CAD build for the part. Positions are in the model's coordinates, mm. Face numbers are marked on the shaded views. A direction names the side the tool comes from. Give positions to 0.01 mm unless a question says otherwise; leave off trailing zeros. Order: outer loops, then holes, each group sorted by start corner. A loop starts at its lowest first (then second) coordinate and runs counter-clockwise, first axis right, second up. Notation, with made-up numbers: M -14,60 L -3,60 A23 ccw -3,96 Z; hole C -39.5,-33 d1. An arc over 180 degrees is marked long. Put each result on its own line as item: value. Start each with the question number.
1) Pin check, flat tips, straight feed: pin 1 (2.5 mm diameter, centred on x = 26, z = 0, fed in from -Y); pin 2 (10.5 mm diameter, centred on x = -23.5, z = 19.5, fed in from +Y); pin 3 (2.5 mm diameter, centred on x = -6.5, y = 1, fed in from +Z); pin 4 (2.5 mm diameter, centred on x = -5, y = 1.5, fed in from -Z). Stop position of each tip, or through.
2) Drill centre lines: line 1 (X direction, y = 9, z = 21); line 2 (Z direction, x = 22.5, y = 6.75); line 3 (X direction, y = 4, z = 12.5). Where is each one in solid material? Low to high. Write a range as [from, to].
3) Cut at C-C (z = -4.5). Write the cut outline in (x, y), and give its area (3 significant figures).
4) Cut at A-A (x = 26). Write the cut outline in (y, z), and give its area (3 significant figures).
5) Cut at D-D (y = 1.75). Write the cut outline in (x, z), and give its area (3 significant figures).
6) Cut at B-B (y = 7.75). Write the cut outline in (x, z), and give its area (3 significant figures).
7) Two-plate mould, pull along Z, no slides. Class the marked faces 1, 2, 3 and 4: released by +Z, released by -Z, zero draft, split by the parting line, or undercut.
8) Tool access for the marked faces 5, 6, 7 and 8: list every direction of +Z, -Z, +X, -X, +Y, -Y with a clear straight run to the whole face (end or side of a thin tool).
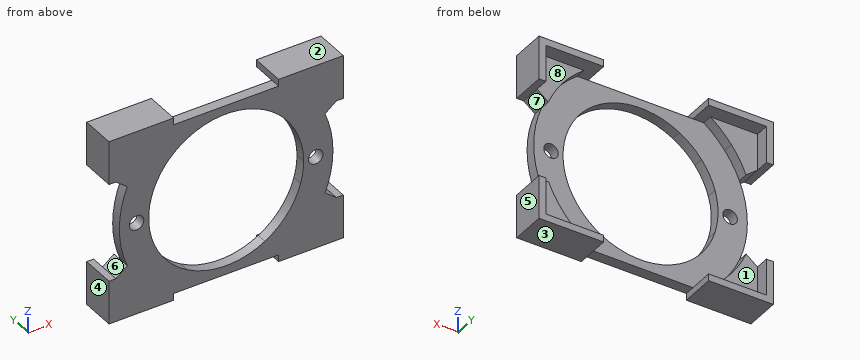
```python
from build123d import *

# Parameters (mm, degrees)
BOSS_EXTRUDE1_DEPTH   = 10
BOSS_EXTRUDE1_2_DEPTH = 10
BOSS_EXTRUDE1_3_DEPTH = 10
BOSS_EXTRUDE1_4_DEPTH = 10
SKETCH1_9_R           = 2.1
BOSS_EXTRUDE2_DEPTH   = 3
BOSS_EXTRUDE3_DEPTH   = 6


with BuildPart() as part:
    # Sketch1 → Boss-Extrude1 (new body)
    with BuildSketch(Plane(origin=(0, 0, 0), x_dir=(1, 0, 0), z_dir=(0, 1, 0))):
        Polygon((-15.231546212, -27), (-15.231546212, -25), (-18.33030278, -25), (-32, -25), (-32, -14.320549047), (-34, -14.320549047), (-34, -27), align=None)
    extrude(amount=BOSS_EXTRUDE1_DEPTH)



with BuildPart() as body_2:
    # Sketch1 → Boss-Extrude1 2 (new body)
    with BuildSketch(Plane(origin=(0, 0, 0), x_dir=(1, 0, 0), z_dir=(0, 1, 0))):
        Polygon((32, -14.320549047), (32, -25), (18.33030278, -25), (15.231546212, -25), (15.231546212, -27), (34, -27), (34, -14.320549047), align=None)
    extrude(amount=BOSS_EXTRUDE1_2_DEPTH)


with BuildPart() as body_3:
    # Sketch1 → Boss-Extrude1 3 (new body)
    with BuildSketch(Plane(origin=(0, 0, 0), x_dir=(1, 0, 0), z_dir=(0, 1, 0))):
        Polygon((32, 25), (32, 14.320549047), (34, 14.320549047), (34, 27), (15.231546212, 27), (15.231546212, 25), (18.33030278, 25), align=None)
    extrude(amount=BOSS_EXTRUDE1_3_DEPTH)


with BuildPart() as body_4:
    # Sketch1 → Boss-Extrude1 4 (new body)
    with BuildSketch(Plane(origin=(0, 0, 0), x_dir=(1, 0, 0), z_dir=(0, 1, 0))):
        Polygon((-18.33030278, 25), (-15.231546212, 25), (-15.231546212, 27), (-34, 27), (-34, 14.320549047), (-32, 14.320549047), (-32, 25), align=None)
    extrude(amount=BOSS_EXTRUDE1_4_DEPTH)


with BuildPart() as part_1:
    add(part.part)

    add(body_2.part)  # Boss-Extrude2 merges body 2

    add(body_3.part)  # Boss-Extrude2 merges body 3

    add(body_4.part)  # Boss-Extrude2 merges body 4
    # Sketch1_9 → Boss-Extrude2 (add)
    # profile 1 of 14: a face of its own
    with BuildSketch(Plane(origin=(0, 0, 0), x_dir=(1, 0, 0), z_dir=(0, 1, 0))):
        with BuildLine():
            Line((-32, 25), (-32, 14.320549047))
            Line((-32, 14.320549047), (-28.692414075, 11.736497543))
            ThreePointArc((-28.692414075, 11.736497543), (-24.428755585, 19.084965301), (-18.33030278, 25))
            Line((-18.33030278, 25), (-32, 25))
        make_face()
    # profile 2 of 14: a face of its own
    with BuildSketch(Plane(origin=(0, 0, 0), x_dir=(1, 0, 0), z_dir=(0, 1, 0))):
        with BuildLine():
            Line((-28.692414075, 11.736497543), (-21.624662992, 6.21481701))
            ThreePointArc((-21.624662992, 6.21481701), (-17.730548409, 13.851990944), (-11.262551698, 19.478319467))
            Line((-11.262551698, 19.478319467), (-18.33030278, 25))
            ThreePointArc((-18.33030278, 25), (-24.428755585, 19.084965301), (-28.692414075, 11.736497543))
        make_face()
    # profile 3 of 14: a face of its own
    with BuildSketch(Plane(origin=(0, 0, 0), x_dir=(1, 0, 0), z_dir=(0, 1, 0))):
        with BuildLine():
            Line((11.262551698, 19.478319467), (18.33030278, 25))
            Line((18.33030278, 25), (15.231546212, 25))
            Line((15.231546212, 25), (-15.231546212, 25))
            Line((-15.231546212, 25), (-18.33030278, 25))
            Line((-18.33030278, 25), (-11.262551698, 19.478319467))
            ThreePointArc((-11.262551698, 19.478319467), (0, 22.5), (11.262551698, 19.478319467))
        make_face()
    # profile 4 of 14: a face of its own
    with BuildSketch(Plane(origin=(0, 0, 0), x_dir=(1, 0, 0), z_dir=(0, 1, 0))):
        with BuildLine():
            Line((21.624662992, 6.21481701), (28.692414075, 11.736497543))
            ThreePointArc((28.692414075, 11.736497543), (24.428755585, 19.084965301), (18.33030278, 25))
            Line((18.33030278, 25), (11.262551698, 19.478319467))
            ThreePointArc((11.262551698, 19.478319467), (17.730548409, 13.851990944), (21.624662992, 6.21481701))
        make_face()
    # profile 5 of 14: a face of its own
    with BuildSketch(Plane(origin=(0, 0, 0), x_dir=(1, 0, 0), z_dir=(0, 1, 0))):
        with BuildLine():
            Line((28.692414075, 11.736497543), (32, 14.320549047))
            Line((32, 14.320549047), (32, 25))
            Line((32, 25), (18.33030278, 25))
            ThreePointArc((18.33030278, 25), (24.428755585, 19.084965301), (28.692414075, 11.736497543))
        make_face()
    # profile 6 of 14: a face of its own
    with BuildSketch(Plane(origin=(0, 0, 0), x_dir=(1, 0, 0), z_dir=(0, 1, 0))):
        with BuildLine():
            Line((21.624662992, -6.21481701), (28.692414075, -11.736497543))
            ThreePointArc((28.692414075, -11.736497543), (31, 0), (28.692414075, 11.736497543))
            Line((28.692414075, 11.736497543), (21.624662992, 6.21481701))
            ThreePointArc((21.624662992, 6.21481701), (22.280091083, 3.138079243), (22.5, 0))
            ThreePointArc((22.5, 0), (22.280091083, -3.138079243), (21.624662992, -6.21481701))
        make_face()
        with Locations(Location((26, 0, 0), (0, 0, 270))):
            Circle(SKETCH1_9_R, mode=Mode.SUBTRACT)
    # profile 7 of 14: a face of its own
    with BuildSketch(Plane(origin=(0, 0, 0), x_dir=(1, 0, 0), z_dir=(0, 1, 0))):
        with BuildLine():
            Line((-24.428755585, -19.084965301), (-17.730548409, -13.851990944))
            ThreePointArc((-17.730548409, -13.851990944), (-20.044694374, -10.220578627), (-21.624662992, -6.21481701))
            Line((-21.624662992, -6.21481701), (-28.692414075, -11.736497543))
            ThreePointArc((-28.692414075, -11.736497543), (-26.813516388, -15.557484979), (-24.428755585, -19.084965301))
        make_face()
    # profile 8 of 14: a face of its own
    with BuildSketch(Plane(origin=(0, 0, 0), x_dir=(1, 0, 0), z_dir=(0, 1, 0))):
        with BuildLine():
            Line((-28.692414075, -11.736497543), (-21.624662992, -6.21481701))
            ThreePointArc((-21.624662992, -6.21481701), (-22.5, 0), (-21.624662992, 6.21481701))
            Line((-21.624662992, 6.21481701), (-28.692414075, 11.736497543))
            ThreePointArc((-28.692414075, 11.736497543), (-31, 0), (-28.692414075, -11.736497543))
        make_face()
        with Locations(Location((-26, 0, 0), (0, 0, 270))):
            Circle(SKETCH1_9_R, mode=Mode.SUBTRACT)
    # profile 9 of 14: a face of its own
    with BuildSketch(Plane(origin=(0, 0, 0), x_dir=(1, 0, 0), z_dir=(0, 1, 0))):
        with BuildLine():
            Line((-32, -14.320549047), (-32, -25))
            Line((-32, -25), (-24.428755585, -19.084965301))
            ThreePointArc((-24.428755585, -19.084965301), (-26.813516388, -15.557484979), (-28.692414075, -11.736497543))
            Line((-28.692414075, -11.736497543), (-32, -14.320549047))
        make_face()
    # profile 10 of 14: a face of its own
    with BuildSketch(Plane(origin=(0, 0, 0), x_dir=(1, 0, 0), z_dir=(0, 1, 0))):
        with BuildLine():
            Line((-32, -25), (-18.33030278, -25))
            ThreePointArc((-18.33030278, -25), (-21.583122502, -22.252389154), (-24.428755585, -19.084965301))
            Line((-24.428755585, -19.084965301), (-32, -25))
        make_face()
    # profile 11 of 14: a face of its own
    with BuildSketch(Plane(origin=(0, 0, 0), x_dir=(1, 0, 0), z_dir=(0, 1, 0))):
        with BuildLine():
            Line((-18.33030278, -25), (-11.262551698, -19.478319467))
            ThreePointArc((-11.262551698, -19.478319467), (-14.766985359, -16.976046165), (-17.730548409, -13.851990944))
            Line((-17.730548409, -13.851990944), (-24.428755585, -19.084965301))
            ThreePointArc((-24.428755585, -19.084965301), (-21.583122502, -22.252389154), (-18.33030278, -25))
        make_face()
    # profile 12 of 14: a face of its own
    with BuildSketch(Plane(origin=(0, 0, 0), x_dir=(1, 0, 0), z_dir=(0, 1, 0))):
        with BuildLine():
            Line((15.231546212, -25), (18.33030278, -25))
            Line((18.33030278, -25), (11.262551698, -19.478319467))
            ThreePointArc((11.262551698, -19.478319467), (0, -22.5), (-11.262551698, -19.478319467))
            Line((-11.262551698, -19.478319467), (-18.33030278, -25))
            Line((-18.33030278, -25), (-15.231546212, -25))
            Line((-15.231546212, -25), (15.231546212, -25))
        make_face()
    # profile 13 of 14: a face of its own
    with BuildSketch(Plane(origin=(0, 0, 0), x_dir=(1, 0, 0), z_dir=(0, 1, 0))):
        with BuildLine():
            Line((11.262551698, -19.478319467), (18.33030278, -25))
            ThreePointArc((18.33030278, -25), (24.428755585, -19.084965301), (28.692414075, -11.736497543))
            Line((28.692414075, -11.736497543), (21.624662992, -6.21481701))
            ThreePointArc((21.624662992, -6.21481701), (17.730548409, -13.851990944), (11.262551698, -19.478319467))
        make_face()
    # profile 14 of 14: a face of its own
    with BuildSketch(Plane(origin=(0, 0, 0), x_dir=(1, 0, 0), z_dir=(0, 1, 0))):
        with BuildLine():
            Line((18.33030278, -25), (32, -25))
            Line((32, -25), (32, -14.320549047))
            Line((32, -14.320549047), (28.692414075, -11.736497543))
            ThreePointArc((28.692414075, -11.736497543), (24.428755585, -19.084965301), (18.33030278, -25))
        make_face()
    extrude(amount=BOSS_EXTRUDE2_DEPTH)

    # Sketch1_11 → Boss-Extrude3 (add)
    with BuildSketch(Plane(origin=(0, 0, 0), x_dir=(1, 0, 0), z_dir=(0, 1, 0))):
        with BuildLine():
            Line((-32, 25), (-32, 14.320549047))
            Line((-32, 14.320549047), (-28.692414075, 11.736497543))
            ThreePointArc((-28.692414075, 11.736497543), (-24.428755585, 19.084965301), (-18.33030278, 25))
            Line((-18.33030278, 25), (-32, 25))
        make_face()
        with BuildLine():
            Line((28.692414075, 11.736497543), (32, 14.320549047))
            Line((32, 14.320549047), (32, 25))
            Line((32, 25), (18.33030278, 25))
            ThreePointArc((18.33030278, 25), (24.428755585, 19.084965301), (28.692414075, 11.736497543))
        make_face()
        with BuildLine():
            Line((18.33030278, -25), (32, -25))
            Line((32, -25), (32, -14.320549047))
            Line((32, -14.320549047), (28.692414075, -11.736497543))
            ThreePointArc((28.692414075, -11.736497543), (24.428755585, -19.084965301), (18.33030278, -25))
        make_face()
        with BuildLine():
            Line((-32, -14.320549047), (-32, -25))
            Line((-32, -25), (-24.428755585, -19.084965301))
            ThreePointArc((-24.428755585, -19.084965301), (-26.813516388, -15.557484979), (-28.692414075, -11.736497543))
            Line((-28.692414075, -11.736497543), (-32, -14.320549047))
        make_face()
        with BuildLine():
            Line((-32, -25), (-18.33030278, -25))
            ThreePointArc((-18.33030278, -25), (-21.583122502, -22.252389154), (-24.428755585, -19.084965301))
            Line((-24.428755585, -19.084965301), (-32, -25))
        make_face()
    extrude(amount=BOSS_EXTRUDE3_DEPTH)


solid = part_1.part
```
Solution:
1. pin 1: through
1. pin 2: y = 6
1. pin 3: z = 25
1. pin 4: z = -25
2. line 1: [-34, -32], [32, 34]
2. line 2: [-27, -25], [25, 27]
2. line 3: [-29.67, -28.37], [28.37, 29.67]
3. outline: M -30.67,0 L -22.05,0 L -22.05,3 L -30.67,3 Z; M 22.05,0 L 30.67,0 L 30.67,3 L 22.05,3 Z
3. area: 51.8 mm²
4. outline: M 0,-27 L 10,-27 L 10,-25 L 6,-25 L 6,-16.88 L 3,-16.88 L 3,-2.1 L 0,-2.1 Z; M 0,2.1 L 3,2.1 L 3,16.88 L 6,16.88 L 6,25 L 10,25 L 10,27 L 0,27 Z
4. area: 226 mm²
5. outline: M -34,-27 L -15.23,-27 L -15.23,-25 L 15.23,-25 L 15.23,-27 L 34,-27 L 34,-14.32 L 32,-14.32 L 28.69,-11.74 A31 ccw 28.69,11.74 L 32,14.32 L 34,14.32 L 34,27 L 15.23,27 L 15.23,25 L -15.23,25 L -15.23,27 L -34,27 L -34,14.32 L -32,14.32 L -28.69,11.74 A31 ccw -28.69,-11.74 L -32,-14.32 L -34,-14.32 Z; hole C -26,0 d4.2; hole C 0,0 d45; hole C 26,0 d4.2
5. area: 1,720 mm²
6. outline: M -34,-27 L -15.23,-27 L -15.23,-25 L -32,-25 L -32,-14.32 L -34,-14.32 Z; M -34,14.32 L -32,14.32 L -32,25 L -15.23,25 L -15.23,27 L -34,27 Z; M 15.23,-27 L 34,-27 L 34,-14.32 L 32,-14.32 L 32,-25 L 15.23,-25 Z; M 15.23,25 L 32,25 L 32,14.32 L 34,14.32 L 34,27 L 15.23,27 Z
6. area: 236 mm²
7. face 1: undercut
7. face 2: released by +Z
7. face 3: released by -Z
7. face 4: zero draft
8. face 5: +Z, -Z, +X, +Y, -Y
8. face 6: -X, +Y, -Y
8. face 7: +X, +Y, -Y
8. face 8: +Y
